```python
from build123d import *

# Parameters (mm, degrees)
F0_W     = 130
F0_H     = 155
F1_DEPTH = 4
F2_R     = 10
F4_DEPTH = 140
F5_R     = 5
F6_R     = 1
F7_R     = 1
F9_D     = 14
F11_D    = 11


# Not quite as in the source:
# - a feature names something its author has since deleted; it is built from what else it names


with BuildPart() as f1:
    # F0 (on Top) → F1 (new body)
    with BuildSketch(Plane.XY):
        with Locations((-65, 36.8233056366)):
            Rectangle(F0_W, F0_H)
    extrude(amount=F1_DEPTH)

    # F2
    f2_edges = [f1.edges().sort_by_distance(p)[0] for p in [
        (0, -40.676694, 2),
        (0, 114.323306, 2),
        (-130, 114.323306, 2),
        (-130, -40.676694, 2),
    ]]
    fillet(f2_edges, radius=F2_R)

    # F3 (on face) → F4 (join)
    with BuildSketch(Plane.XY.offset(4)):
        Polygon((-16, 26.8233056366), (-16, 61.8233056366), (-114, 61.8233056366), (-114, 26.8233056366), (-111.5, 26.8233056366), (-111.5, 59.3233056366), (-18.5, 59.3233056366), (-18.5, 26.8233056366), align=None)
    extrude(amount=F4_DEPTH)

    # F5
    f5_edges = [f1.edges().sort_by_distance(p)[0] for p in [
        (-114, 61.823306, 74),
        (-16, 61.823306, 74),
    ]]
    fillet(f5_edges, radius=F5_R)

    # F6
    f6_edges = [f1.edges().sort_by_distance(p)[0] for p in [
        (-18.5, 59.323306, 74),
        (-111.5, 59.323306, 74),
    ]]
    fillet(f6_edges, radius=F6_R)

    # F7
    f7_edges = [f1.edges().sort_by_distance(p)[0] for p in [
        (-112.75, 26.823306, 144),
        (-17.25, 26.823306, 144),
    ]]
    fillet(f7_edges, radius=F7_R)

    # F9 (through all)
    with Locations(Plane.XY.offset(4)):
        with Locations((-22.5, 91.8233056366), (-65, 91.8233056366), (-107.5, 91.8233056366)):
            Hole(F9_D / 2)

    # F11 (through all)
    with Locations(Plane(origin=(0, 61.8233056366, 0), x_dir=(-1, 0, 0), z_dir=(0, 1, 0))):
        with Locations((42.5, 43.8), (87.5, 43.8), (42.5, 120), (87.5, 120)):
            Hole(F11_D / 2)


solid = f1.part
```
For this review, take the finished solid that the model builds, in its own axes (mm). A direction names the side the tool comes from. Give positions to 0.01 mm unless a question says otherwise; leave off trailing zeros. Write each loop counter-clockwise with the first axis right and the second up, starting at its lowest first coordinate (ties: lowest second). Pieces come first, ordered by that corner, then holes.
Item 1: Machinability: for faces 4 (the face through (-112.496, 60.398, 74.98)), 5 (the face through (-18.5, 43, 73)), 6 (the face through (-64, 61.823, 73)), which of the approach directions +Z, -Z, +X, -X, +Y, -Y give a long, thin tool a straight path to every point of the face, cutting with its end or side? Answer none if there is none.
Item 2: Take a section at B-B (x = -42.5). Give the boundary of the cut face in (y, z), and give its area (3 significant figures).
Item 3: Insertion check: P1, Ø3, axis at x = -17.5, z = 54.5, coming from the -Y side; P2, Ø8.5, axis at x = -107.5, y = 91.82, coming from the -Z side; P3, Ø8, axis at x = -61.5, z = 122, coming from the -Y side; P4, Ø16, axis at y = 40.5, z = 87.5, coming from the -X side. Each pin has a flat end and moves straight along its axis. Give the tip position at first contact, or say it passes through.
Item 4: Take a section at A-A (z = 43.8). Give the boundary of the cut face in (x, y), and give its area (3 significant figures).
Item 5: The part is to be moulded in two halves that separate along Y. For faces 1 (the face through (-130, 36, 2)), 2 (the face through (-66, -40.677, 2)), 3 (the face through (-64.089, 98.764, 1.972)), say which applies: +Y half, -Y half, draft (parallel to the pull), parting line (faces both ways), or undercut.
Item 6: Wall thickness on probe 1 along Y at (x, z) = (-107.5, 1.55); probe 2 along X at (y, z) = (36, 91); probe 3 along Z at (x, y) = (-45, 64.5): over which ranges is each line inside the solid? List them lowest first.
Item 7: Take a section at C-C (y = 39.5). Give the boundary of the cut face in (x, z), and give its area (3 significant figures).
Item 8: Take a section at D-D (x = -105.5). Give the boundary of the cut face in (y, z), and give its area (3 significant figures).
Established:
1. face 4: +Z, -X, +Y
1. face 5: +Z, -Y
1. face 6: +Z, +X, -X, +Y
2. outline: (-40.68, 0) - (114.32, 0) - (114.32, 4) - (61.82, 4) - (61.82, 38.3) - (59.32, 38.3) - (59.32, 4) - (-40.68, 4) - close; (59.32, 49.3) - (61.82, 49.3) - (61.82, 114.5) - (59.32, 114.5) - close; (59.32, 125.5) - (61.82, 125.5) - (61.82, 144) - (59.32, 144) - close
2. area: 915 mm2
3. P1: stops at y = 26.82
3. P2: passes through
3. P3: stops at y = 59.32
3. P4: stops at x = -114
4. outline: (-114, 26.82) - (-111.5, 26.82) - (-111.5, 58.32) arc R1 cw to (-110.5, 59.32) - (-93, 59.32) - (-93, 61.82) - (-109, 61.82) arc R5 ccw to (-114, 56.82) - close; (-82, 59.32) - (-48, 59.32) - (-48, 61.82) - (-82, 61.82) - close; (-37, 59.32) - (-19.5, 59.32) arc R1 cw to (-18.5, 58.32) - (-18.5, 26.82) - (-16, 26.82) - (-16, 56.82) arc R5 ccw to (-21, 61.82) - (-37, 61.82) - close
4. area: 342 mm2
5. face 1: draft
5. face 2: -Y half
5. face 3: undercut
6. probe 1: y = -40.68 to 84.82, 98.82 to 114.32
6. probe 2: x = -114 to -111.5, -18.5 to -16
6. probe 3: z = 0 to 4
7. outline: (-130, 0) - (0, 0) - (0, 4) - (-16, 4) - (-16, 144) - (-18.5, 144) - (-18.5, 4) - (-111.5, 4) - (-111.5, 144) - (-114, 144) - (-114, 4) - (-130, 4) - close
7. area: 1,220 mm2
8. outline: (-40.68, 0) - (85.12, 0) - (85.12, 4) - (61.82, 4) - (61.82, 144) - (59.32, 144) - (59.32, 4) - (-40.68, 4) - close; (98.53, 0) - (114.32, 0) - (114.32, 4) - (98.53, 4) - close
8. area: 916 mm2
